```python
from build123d import *

# Parameters (mm, degrees)
BASPROSKE_W        = 10
BASPROSKE_H        = 23.625
TOOTHCUT_DEPTH     = 35.875224014
TEETHCUTS_COUNT    = 25
TEETHCUTS_ANGLE    = 345.6
BORSKE_R           = 4
BORE_DEPTH         = 50.0000508
SKETCH1_R          = 11
CUT_EXTRUDE1_DEPTH = 7
CUT_EXTRUDE2_REACH = 36.122
SKETCH2_R          = 8
CUT_EXTRUDE3_REACH = 36.862
SKETCH3_R          = 1.6
CIRPATTERN1_COUNT  = 6
CHAMFER1_SIZE      = 0.5


with BuildPart() as part:
    # BasProSke → Base-Revolve (revolve)
    with BuildSketch(Plane(origin=(0, 0, 0), x_dir=(1, 0, 0), z_dir=(0, 1, 0)), mode=Mode.PRIVATE) as base_revolve_sk:
        with Locations((5, 11.8125)):
            Rectangle(BASPROSKE_W, BASPROSKE_H)
    revolve(base_revolve_sk.sketch.rotate(Axis((-10, 0, 0), (1, 0, 0)), 180), axis=Axis((-10, 0, 0), (1, 0, 0)))

    # TooCutSke → ToothCut (cut, through all)
    with BuildSketch(Plane(origin=(0, 0, 0), x_dir=(0, 0, -1), z_dir=(1, 0, 0))):
        with BuildLine():
            ThreePointArc((0.818998709, 19.669456611), (0, 19.6865), (-0.818998709, 19.669456611))
            ThreePointArc((-0.818998709, 19.669456611), (-1.409254574, 21.695516899), (-2.467415344, 23.521336732))
            ThreePointArc((-2.467415344, 23.521336732), (0, 23.6504), (2.467415344, 23.521336732))
            ThreePointArc((2.467415344, 23.521336732), (1.409254574, 21.695516899), (0.818998709, 19.669456611))
        make_face()
    toothcut = extrude(amount=TOOTHCUT_DEPTH, mode=Mode.SUBTRACT)

    # TeethCuts: ToothCut ×25 about axis
    teethcuts_axis = Axis((-10, 0, 0), (1, 0, 0))
    for i in range(1, TEETHCUTS_COUNT):
        add(toothcut.rotate(teethcuts_axis, i * TEETHCUTS_ANGLE / (TEETHCUTS_COUNT - 1)), mode=Mode.SUBTRACT)

    # BorSke → Bore (cut, symmetric)
    with BuildSketch(Plane(origin=(0, 0, 0), x_dir=(0, 0, -1), z_dir=(1, 0, 0))):
        with Locations(Location((0, 0, 0), (0, 0, 180))):
            Circle(BORSKE_R)
    extrude(amount=BORE_DEPTH, both=True, mode=Mode.SUBTRACT)

    # Sketch1 → Cut-Extrude1 (cut)
    with BuildSketch(Plane(origin=(10, 0, 0), x_dir=(0, 0, -1), z_dir=(1, 0, 0))):
        Circle(SKETCH1_R)
    extrude(amount=-CUT_EXTRUDE1_DEPTH, mode=Mode.SUBTRACT)

    # Sketch2 → Cut-Extrude2 (cut, up to next)
    with BuildSketch(Plane(origin=(3, 0, 0), x_dir=(0, 0, -1), z_dir=(1, 0, 0)), mode=Mode.PRIVATE) as cut_extrude2_sk1:
        Circle(SKETCH2_R)
    cut_extrude2_tool1 = extrude(cut_extrude2_sk1.sketch, amount=-CUT_EXTRUDE2_REACH, mode=Mode.PRIVATE) & part.part
    add(cut_extrude2_tool1.solids().sort_by_distance((3, 0, 0))[0], mode=Mode.SUBTRACT)

    # Sketch3 → Cut-Extrude3 (cut, up to next)
    with BuildSketch(Plane(origin=(10, 0, 0), x_dir=(0, 0, -1), z_dir=(1, 0, 0)), mode=Mode.PRIVATE) as cut_extrude3_sk1:
        with Locations((0, 15)):
            Circle(SKETCH3_R)
    cut_extrude3_tool1 = extrude(cut_extrude3_sk1.sketch, amount=-CUT_EXTRUDE3_REACH, mode=Mode.PRIVATE) & part.part
    cut_extrude3 = cut_extrude3_tool1.solids().sort_by_distance((10, 15, 0))[0]
    add(cut_extrude3, mode=Mode.SUBTRACT)

    # CirPattern1: Cut-Extrude3 ×6 about axis
    cirpattern1_axis = Axis((0, 0, 0), (1, 0, 0))
    for i in range(1, CIRPATTERN1_COUNT):
        add(cut_extrude3.rotate(cirpattern1_axis, i * 360 / CIRPATTERN1_COUNT), mode=Mode.SUBTRACT)

    # Chamfer1
    chamfer1_edges = [part.edges().sort_by_distance(p)[0] for p in [
        (10, 0, 11),
        (3, 0, 8),
        (0, 0, 8),
    ]]
    chamfer(chamfer1_edges, length=CHAMFER1_SIZE)


solid = part.part
```
CAD build for the part. Positions are in the model's coordinates, mm. A direction names the side the tool comes from. Coordinates: 2 decimals unless noted, no trailing zeros. Return JSON: item names as keys, results as strings. Group by question number.
Q1. Drill centre lines: line 1 (Y direction, x = 1.25, z = 0) (1 decimal); line 2 (Y direction, x = 6, z = 0) (1 decimal); line 3 (Z direction, x = 7, y = 0.5). Where is each one in solid material? Low to high.
Q2. Which spindle directions (+Z, -Z, +X, -X, +Y, -Y) get a long thin tool onto all of the face, cutting with end or side? Do faces 1 (the face through (4.93, -3.7, -19.336)), 2 (the face through (4.93, 19.686, -0.011)), 3 (the face through (4.93, 14.343, -13.485)). Say none if no direction does.
Q3. Cut at A-A, the plane x = 4.25. State how many separate pieces and enclosed holes the cut face has, then the cut area to 3 significant figures.
Q4. Pull direction Z, two halves, no side cores. Call faces 4 (the face through (4.93, -5.46, -21.06)), 5 (the face through (4.93, 8.054, 20.209)), 6 (the face through (4.93, 18.342, -11.698)), 7 (the face through (4.93, 17.25, -9.49)): released by +Z, released by -Z, zero draft, split by the parting line, or undercut.
Q5. Flat gauge pins, fed straight in: pin 1 (2 mm diameter, centred on x = 9, z = 3.5, fed in from -Y); pin 2 (11 mm diameter, centred on y = -0.5, z = -4, fed in from +X); pin 3 (1.9 mm diameter, centred on y = -7.5, z = 12.99, fed in from +X); pin 4 (6 mm diameter, centred on x = 3, y = 17, fed in from +Z). Where does each tip first touch, or does it go through?
Returned:
{
 "1": {"line 1": "y = -23.6 to -16.6, -13.4 to -8, 8 to 13.4, 16.6 to 19.7", "line 2": "y = -23.6 to -16.6, -13.4 to -11, 11 to 13.4, 16.6 to 19.7", "line 3": "z = -19.68 to -10.99, 10.99 to 19.68"},
 "2": {"face 1": "-Z, +X, -X", "face 2": "+X, -X, +Y", "face 3": "+X, -X"},
 "3": {"separate pieces": "1", "enclosed holes": "7", "area": "1,040 mm2"},
 "4": {"face 4": "released by -Z", "face 5": "released by +Z", "face 6": "undercut", "face 7": "undercut"},
 "5": {"pin 1": "stops at y = -21.94", "pin 2": "stops at x = 3", "pin 3": "passes through", "pin 4": "stops at z = 18.53"}
}
